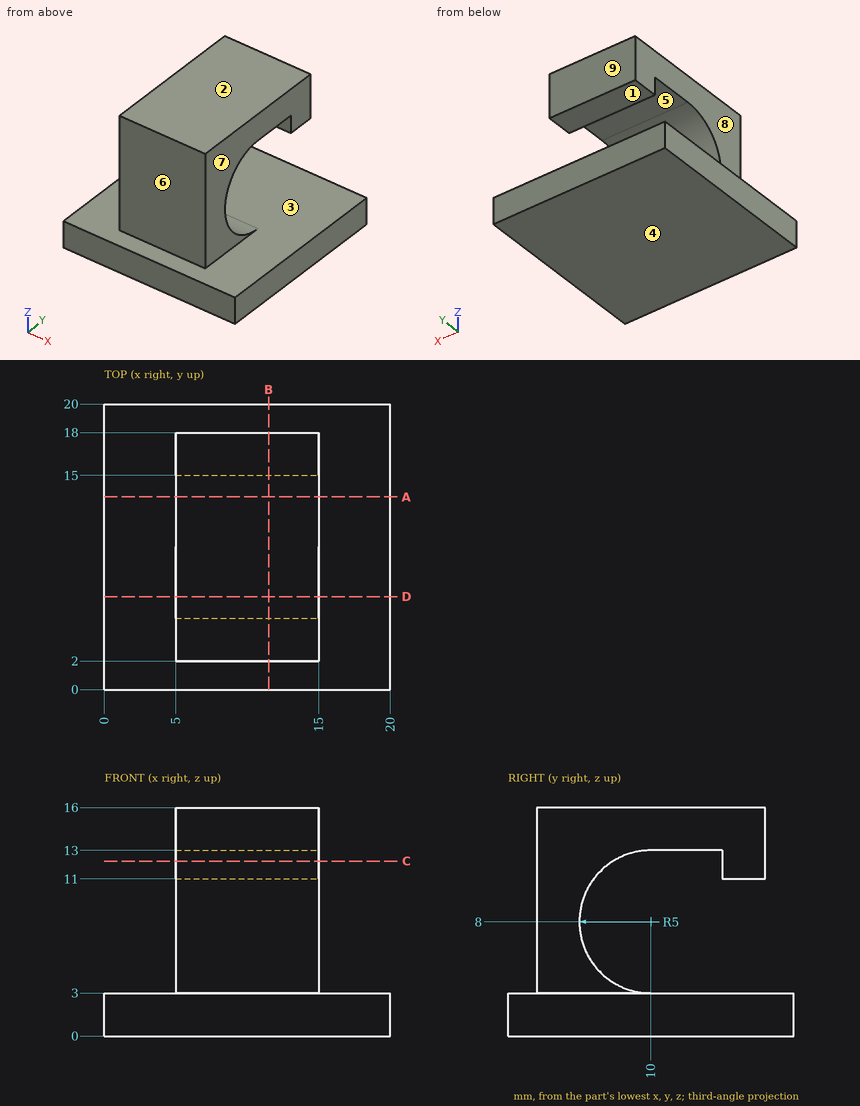
Design review of the part shown in the three views and the two pictorial views. Dimensions are in mm from the part's minimum x, y and z. A direction names the side the tool comes from. Coordinates: 2 decimals unless noted, no trailing zeros. Write each loop counter-clockwise with the first axis right and the second up, starting at its lowest first coordinate (ties: lowest second). Pieces come first, ordered by that corner, then holes.
(1) Add section A-A on y = 13.5. Give the boundary of the cut face in (x, z), then the cut area to 3 significant figures.
(2) For pin 1 Ø8 at (y, z) = (11, 4.5) entering from +X; pin 2 Ø3 at (y, z) = (10, 12) entering from +X; pin 3 Ø4 at (y, z) = (12, 10.5) entering from +X; pin 4 Ø8 at (x, z) = (18, 13) entering from +Y, all flat-tipped, find the tip position at first contact; note any pin that passes through.
(3) Add section B-B on x = 11.5. Give the boundary of the cut face in (y, z), then the cut area to 3 significant figures.
(4) Add section D-D on y = 6.5. Give the boundary of the cut face in (x, z).
(5) Wall thickness on probe 1 along Z at (x, y) = (9.25, 15.25); probe 2 along Z at (x, y) = (17, 17.25); probe 3 along X at (y, z) = (7, 14.5): over which ranges is each line inside the solid? List them lowest first.
(6) Tool access review of the marked faces 5, 6, 7, 8 and 9: name each direction out of +Z, -Z, +X, -X, +Y, -Y from which nothing blocks a thin tool from reaching the whole face with its end or side.
(7) The part is to be moulded in two halves that separate along Z. For the marked faces 1, 2, 3 and 4, say which applies: +Z half, -Z half, draft (parallel to the pull), parting line (faces both ways), or undercut.
(8) Add section C-C on z = 12.25. Give the boundary of the cut face in (x, y), then the cut area to 3 significant figures.
Answer sheet:
1. outline: (0, 0) - (20, 0) - (20, 3) - (0, 3) - close; (5, 13) - (15, 13) - (15, 16) - (5, 16) - close
1. area: 90.0 mm2
2. pin 1: stops at x = 20
2. pin 2: stops at x = 15
2. pin 3: passes through
2. pin 4: stops at y = 18
3. outline: (0, 0) - (20, 0) - (20, 3) - (10, 3) arc R5 cw to (10, 13) - (15, 13) - (15, 11) - (18, 11) - (18, 16) - (2, 16) - (2, 3) - (0, 3) - close
3. area: 155 mm2
4. outline: (0, 0) - (20, 0) - (20, 3) - (15, 3) - (15, 4.43) - (5, 4.43) - (5, 3) - (0, 3) - close; (5, 11.57) - (15, 11.57) - (15, 16) - (5, 16) - close
5. probe 1: z = 0 to 3, 11 to 16
5. probe 2: z = 0 to 3
5. probe 3: x = 5 to 15
6. face 5: +X, -X
6. face 6: +Z, +X, -X, -Y
6. face 7: +Z, +X, +Y, -Y
6. face 8: +Z, -X, +Y, -Y
6. face 9: +Z, +X, -X, +Y
7. face 1: undercut
7. face 2: +Z half
7. face 3: undercut
7. face 4: -Z half
8. outline: (5, 2) - (15, 2) - (15, 7.37) - (5, 7.37) - close; (5, 15) - (15, 15) - (15, 18) - (5, 18) - close
8. area: 83.7 mm2
